Input: part model. Units: mm. Frame: model coordinates. Face numbers are marked on the shaded views. A direction names the side the tool comes from. Give positions to 0.01 mm unless a question says otherwise; leave off trailing zeros. Order: outer loops, then holes, each group sorted by start corner. A loop starts at its lowest first (then second) coordinate and runs counter-clockwise, first axis right, second up. Notation, with made-up numbers: (-33.5, -37.75) - (24.5, -37.75) arc R20 cw to (24.5, -13.75) - close; hole circle Ø10 at (78.25, 78). An arc over 180 degrees is marked (long way). Answer in a Markdown table with one row per item. Add a question column.
from build123d import *

# Parameters (mm, degrees)
F1_DEPTH = 63.5
F2_DEPTH = 25.4
F3_DEPTH = 12.7
F5_R     = 6.35


with BuildPart() as f1:
    # F0 (on Front) → F1 (new body, symmetric)
    with BuildSketch(Plane.XZ):
        Polygon((-41.275, 9.525), (-41.275, -9.525), (41.275, -9.525), (41.275, 9.525), (22.225, 9.525), align=None)
    extrude(amount=F1_DEPTH, both=True)

    # F0 (on Front) → F2 (join, symmetric)
    with BuildSketch(Plane.XZ):
        with BuildLine():
            Line((22.225, 9.525), (41.275, 9.525))
            Line((41.275, 9.525), (41.275, 27.051))
            ThreePointArc((41.275, 27.051), (45.9246798487, 38.2763201513), (57.15, 42.926))
            Line((57.15, 42.926), (60.325, 42.926))
            Line((60.325, 42.926), (60.325, 61.976))
            Line((60.325, 61.976), (57.15, 61.976))
            ThreePointArc((57.15, 61.976), (32.4542956671, 51.7467043329), (22.225, 27.051))
            Line((22.225, 27.051), (22.225, 9.525))
        make_face()
        Polygon((82.0737038128, 61.976), (60.325, 61.976), (60.325, 42.926), (82.0737038128, 42.926), (85.725, 42.926), (85.725, 61.976), align=None)
    extrude(amount=F2_DEPTH, both=True)

    # F0 (on Front) → F3 (join, symmetric)
    with BuildSketch(Plane.XZ):
        with BuildLine():
            add(Edge.make_bspline(
                [(-41.275, 9.525), (-41.2416942418, 43.5823909938), (19.5547696203, 62.110837549), (57.15, 61.976)],
                knots=[0, 0, 0, 0, 111.5284180198, 111.5284180198, 111.5284180198, 111.5284180198], degree=3))
            Line((-41.275, 9.525), (22.225, 9.525))
            Line((22.225, 9.525), (22.225, 27.051))
            ThreePointArc((22.225, 27.051), (32.4542956671, 51.7467043329), (57.15, 61.976))
        make_face()
    extrude(amount=F3_DEPTH, both=True)

    # F0 (on Front) → F4 (revolve)
    with BuildSketch(Plane.XZ):
        Polygon((111.125, 66.675), (85.725, 66.675), (85.725, 61.976), (85.725, 42.926), (85.725, 38.1), (111.125, 38.1), align=None)
    revolve(axis=Axis((85.725, 0, 52.3875), (0, 0, 1)))

    # F5
    f5_edges = [f1.edges().sort_by_distance(p)[0] for p in [
        (-41.275, -63.5, 0),
        (41.275, -63.5, 0),
        (41.275, 63.5, 0),
        (-41.275, 63.5, 0),
    ]]
    fillet(f5_edges, radius=F5_R)


solid = f1.part
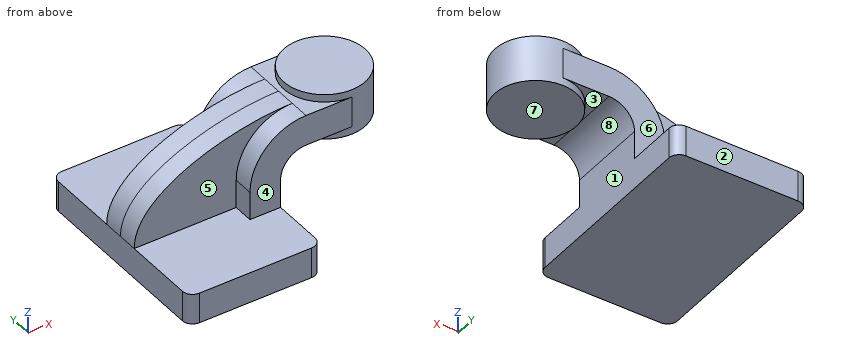
Q1. Access query for the marked faces 4, 5, 6, 7 and 8. Directions: +Z, -Z, +X, -X, +Y, -Y. A direction counts if a zero-diameter tool reaches every point of the face in a straight line with its end or side. Return the directions, or none.
Q2. Section B-B, the plane y = -16.5. Return loops of the section in (x, z) (3 decimals).
Q3. Line query: probe 1 along Z at (x, y) = (-22, 35.5) (3 decimals); probe 2 along Z at (x, y) = (68, 4) (3 decimals); probe 3 along X at (y, z) = (19, 11) (3 decimals). Output: solid intervals per line, ascending.
Q4. Section A-A, the plane z = 2.5. Return loops of the section in (x, y) (3 decimals).
Q5. Section C-C, the plane y = 40.5. Return loops of the section in (x, z) (3 decimals).
Q6. Contact query for flat-ended pins moving along their axis: P1, Ø4, axis at y = -20, z = 16.5, coming from the -X side (3 decimals); P2, Ø8, axis at y = 4.5, z = 0, coming from the +X side (3 decimals); P3, Ø1.5, axis at x = 78, z = 51.5, coming from the +Y side. Output: stop coordinate, or through.
Q7. Pull-direction query (X, two-part tool) for the marked faces 1, 2 and 3; classes: +X half, -X half, draft (parallel to the pull), parting line (faces both ways), or undercut.
Computed:
| question | item | result |
|---|---|---|
| 1 | face 4 | +Z, +X, -X, -Y |
| 1 | face 5 | +Z, -X, -Y |
| 1 | face 6 | +Z, +X, -X, +Y |
| 1 | face 7 | -Z, +X, +Y, -Y |
| 1 | face 8 | -Z, +Y, -Y |
| 2 | outline | (-41.275, -9.525) - (41.275, -9.525) - (41.275, 27.051) arc R15.875 cw to (57.15, 42.926) - (66.414, 42.926) - (66.414, 38.1) - (105.036, 38.1) - (105.036, 66.675) - (66.414, 66.675) - (66.414, 61.976) - (57.15, 61.976) arc R34.925 ccw to (22.225, 27.051) - (22.225, 9.525) - (-41.275, 9.525) - close |
| 3 | probe 1 | z = -9.525 to 9.525 |
| 3 | probe 2 | z = 38.1 to 66.675 |
| 3 | probe 3 | x = 22.225 to 41.275 |
| 4 | outline | (-41.275, -57.15) arc R6.35 ccw to (-34.925, -63.5) - (34.925, -63.5) arc R6.35 ccw to (41.275, -57.15) - (41.275, 57.15) arc R6.35 ccw to (34.925, 63.5) - (-34.925, 63.5) arc R6.35 ccw to (-41.275, 57.15) - close |
| 5 | outline | (-41.275, -9.525) - (41.275, -9.525) - (41.275, 9.525) - (-41.275, 9.525) - close |
| 6 | P1 | stops at x = 22.225 |
| 6 | P2 | stops at x = 41.275 |
| 6 | P3 | stops at y = 25.4 |
| 7 | face 1 | +X half |
| 7 | face 2 | draft |
| 7 | face 3 | undercut |
